Verification items for this drawing (mm, ordinates from the low corner). A direction names the side the tool comes from. Round coordinates to 2 decimals unless told otherwise and drop trailing zeros. Loops run counter-clockwise (first coordinate to the right, second up) from the corner with the lowest first, then second, coordinate; pieces in that order, holes last. Notation, with made-up numbers: M 10.25,79.5 L 44.25,79.5 A22 cw 44.25,86.5 Z; hole C 26.25,-35 d8. An arc over 180 degrees is marked long. Use one line per item in the form item = value. Start each with the question number.
1. Cross-section at D-D (x = 36.5). Record the boundary of the cut face in (y, z).
2. Material ranges on line 1 (Y direction, x = 23, z = 1); line 2 (X direction, y = 33, z = 7); line 3 (Z direction, x = 13, y = 38), recorded low to high.
3. Draft check along Y on the marked faces 6, 7 and 8. Enter one of: pulls with the +Y half, pulls with the -Y half, needs draft (parallel to the pull), parting line crosses it, or undercut.
4. Set-up check for the marked faces 1, 2, 3, 4 and 5: record each of +Z, -Z, +X, -X, +Y, -Y from which the full face is reachable in a straight line by a thin tool's end or side.
5. Cross-section at C-C (y = 32). Record the boundary of the cut face in (x, z), then the cut area to 3 significant figures.
6. Go/stop test with flat-tipped pins: pin 1 (8 mm diameter, centred on x = 21.5, y = 36, fed in from -Z); pin 2 (5 mm diameter, centred on y = 33, z = 13, fed in from +X); pin 3 (8 mm diameter, centred on y = 36, z = 8.5, fed in from -X). Record where each tip stops, or that it passes through.
7. Cross-section at B-B (x = 17.5). Record the boundary of the cut face in (y, z).
8. Cross-section at A-A (z = 10). Record the boundary of the cut face in (x, y).
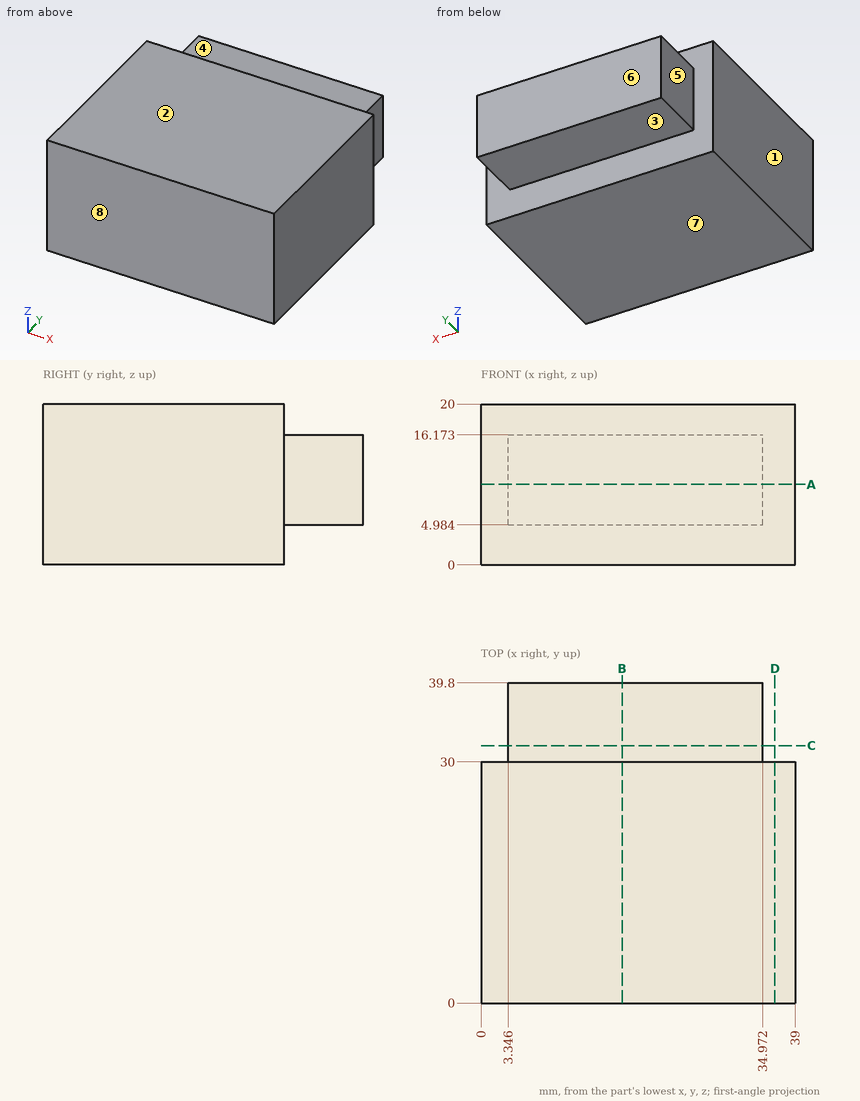
Reported:
q1.outline = M 0,0 L 30,0 L 30,20 L 0,20 Z
q2.line_1 = 0 to 30
q2.line_2 = 3.35 to 34.97
q2.line_3 = 4.98 to 16.17
q3.face_6 = pulls with the +Y half
q3.face_7 = needs draft
q3.face_8 = pulls with the -Y half
q4.face_1 = +Z, -Z, -X, +Y, -Y
q4.face_2 = +Z, +X, -X, +Y, -Y
q4.face_3 = -Z, +X, -X, +Y
q4.face_4 = +Z, +X, -X, +Y
q4.face_5 = +Z, -Z, -X, +Y
q5.outline = M 3.35,4.98 L 34.97,4.98 L 34.97,16.17 L 3.35,16.17 Z
q5.area = 354 mm²
q6.pin_1 = 4.98
q6.pin_2 = 34.97
q6.pin_3 = 3.35
q7.outline = M 0,0 L 30,0 L 30,4.98 L 39.8,4.98 L 39.8,16.17 L 30,16.17 L 30,20 L 0,20 Z
q8.outline = M 0,0 L 39,0 L 39,30 L 34.97,30 L 34.97,39.8 L 3.35,39.8 L 3.35,30 L 0,30 Z
